```python
from build123d import *

# Parameters (mm, degrees)
SKETCH1_R               = 20
BOSS_EXTRUDE1_DEPTH     = 100
SKETCH2_W               = 65
SKETCH2_H               = 9.328019595
SKETCH2_H_2             = 21.34396081
BOSS_EXTRUDE2_DEPTH     = 8
CUT_EXTRUDE2_DEPTH      = 21
CUT_EXTRUDE2_DEPTH_BACK = 21


with BuildPart() as part:
    # Sketch1 → Boss-Extrude1 (new body)
    with BuildSketch(Plane(origin=(0, 0, 0), x_dir=(0, 0, -1), z_dir=(1, 0, 0))):
        Circle(SKETCH1_R)
        with BuildLine():
            Line((-10.671980405, -8), (10.671980405, -8))
            ThreePointArc((10.671980405, -8), (0, 13.337584705), (-10.671980405, -8))
        make_face(mode=Mode.SUBTRACT)
    extrude(amount=-BOSS_EXTRUDE1_DEPTH)

    # Sketch2 → Boss-Extrude2 (add)
    with BuildSketch(Plane(origin=(0, -8, 0), x_dir=(1, 0, 0), z_dir=(0, 1, 0))):
        with Locations((-67.5, 15.335990202)):
            Rectangle(SKETCH2_W, SKETCH2_H)
        with Locations((-67.5, 0)):
            Rectangle(SKETCH2_W, SKETCH2_H_2)
        with Locations((-67.5, -15.335990202)):
            Rectangle(SKETCH2_W, SKETCH2_H)
    extrude(amount=BOSS_EXTRUDE2_DEPTH)

    # Sketch3 → Cut-Extrude2 (cut, two sides)
    with BuildSketch(Plane.XY) as cut_extrude2_sk:
        Polygon((0, 20), (-60, 20), (0, -5), align=None)
    extrude(amount=CUT_EXTRUDE2_DEPTH, mode=Mode.SUBTRACT)
    extrude(cut_extrude2_sk.sketch, amount=-CUT_EXTRUDE2_DEPTH_BACK, mode=Mode.SUBTRACT)


solid = part.part
```
The listing builds one solid part. Answer for the finished solid, in the listing's coordinates (mm). Give positions to 0.01 mm unless a question says otherwise; leave off trailing zeros. Order: outer loops, then holes, each group sorted by start corner. A loop starts at its lowest first (then second) coordinate and runs counter-clockwise, first axis right, second up. Notation, with made-up numbers: (-27, 83) -> (-19, 83) arc R12 ccw to (-19, 104) -> close; hole circle Ø9 at (28, -21). An arc over 180 degrees is marked (long way). One line per item, written item: value.
1) Find section B-B, the plane x = -72. Determine the outline of the cut face in (y, z), plus the area to 3 significant figures.
Reported:
outline: (-8, -20) -> (0, -20) arc R20 ccw to (0, 20) -> (-8, 20) -> (-8, 18.33) arc R20 ccw to (-8, -18.33) -> close; hole (0, -13.34) arc R13.34 ccw to (0, 13.34) -> close
area: 986 mm^2
2) Flat-ended cylindrical pins translate along their axes: P1, Ø1.3, axis at x = -57, z = 19.5, coming from the -Y side; P2, Ø5, axis at x = -45, y = 6, coming from the -Z side; P3, Ø4, axis at y = -2.5, z = -5, coming from the +X side. Find the tip coordinate at first contact, or state that the pin passes through.
Reported:
P1: stops at y = -8
P2: stops at z = -19.69
P3: stops at x = -35
3) Find section D-D, the plane x = -42. Determine the outline of the cut face in (y, z).
Reported:
outline: (-8, -20) -> (0, -20) arc R20 ccw to (12.5, -15.61) -> (12.5, -4.65) arc R13.34 cw to (0, -13.34) -> (0, 13.34) arc R13.34 cw to (12.5, 4.65) -> (12.5, 15.61) arc R20 ccw to (0, 20) -> (-8, 20) -> (-8, 18.33) arc R20 ccw to (-8, -18.33) -> close
4) Find the intervals of material crossed by line 1 (Z direction, x = -23.5, y = 0); line 2 (Y direction, x = -64, z = 0); line 3 (Y direction, x = -24.5, z = 0), in increasing order.
Reported:
line 1: z = -20 to -13.34, 13.34 to 20
line 2: y = -20 to 0, 13.34 to 20
line 3: y = -20 to -8
5) Determine the mould class of faces 1 (the flat face through (-37.087, 10.453, 9.169)), 2 (the flat face through (-68, 0, 0)), 3 (the cylindrical face through (-60.41, 13.33, -0.41)), 4 (the flat face through (-100, -0.3, -0.3)) for opening direction Y: pulls with the +Y half, pulls with the -Y half, needs draft (parallel to the pull), parting line crosses it, or undercut.
Reported:
face 1: pulls with the +Y half
face 2: undercut
face 3: undercut
face 4: needs draft
6) Find section C-C, the plane y = 8.5. Determine the outline of the cut face in (x, z), plus the area to 3 significant figures.
Reported:
outline: (-100, -18.1) -> (-32.4, -18.1) -> (-32.4, -10.28) -> (-100, -10.28) -> close; (-100, 10.28) -> (-32.4, 10.28) -> (-32.4, 18.1) -> (-100, 18.1) -> close
area: 1,060 mm^2
7) Find section A-A, the plane z = -7.5. Determine the outline of the cut face in (x, y).
Reported:
outline: (-100, -18.54) -> (0, -18.54) -> (0, -8) -> (-35, -8) -> (-35, 0) -> (-100, 0) -> close; (-100, 11.03) -> (-38.47, 11.03) -> (-56.5, 18.54) -> (-100, 18.54) -> close
